Design review of the part shown in the three views and the two pictorial views. Dimensions are in mm from the part's minimum x, y and z. A direction names the side the tool comes from. Give positions to 0.01 mm unless a question says otherwise; leave off trailing zeros. Loops run counter-clockwise (first coordinate to the right, second up) from the corner with the lowest first, then second, coordinate; pieces in that order, holes last. Notation, with made-up numbers: M 10,11 L 15,11 A18 ccw 15,23 Z; hole C 37.25,22 d7. An arc over 180 degrees is marked long. Return JSON: item names as keys, results as strings. Group by question number.
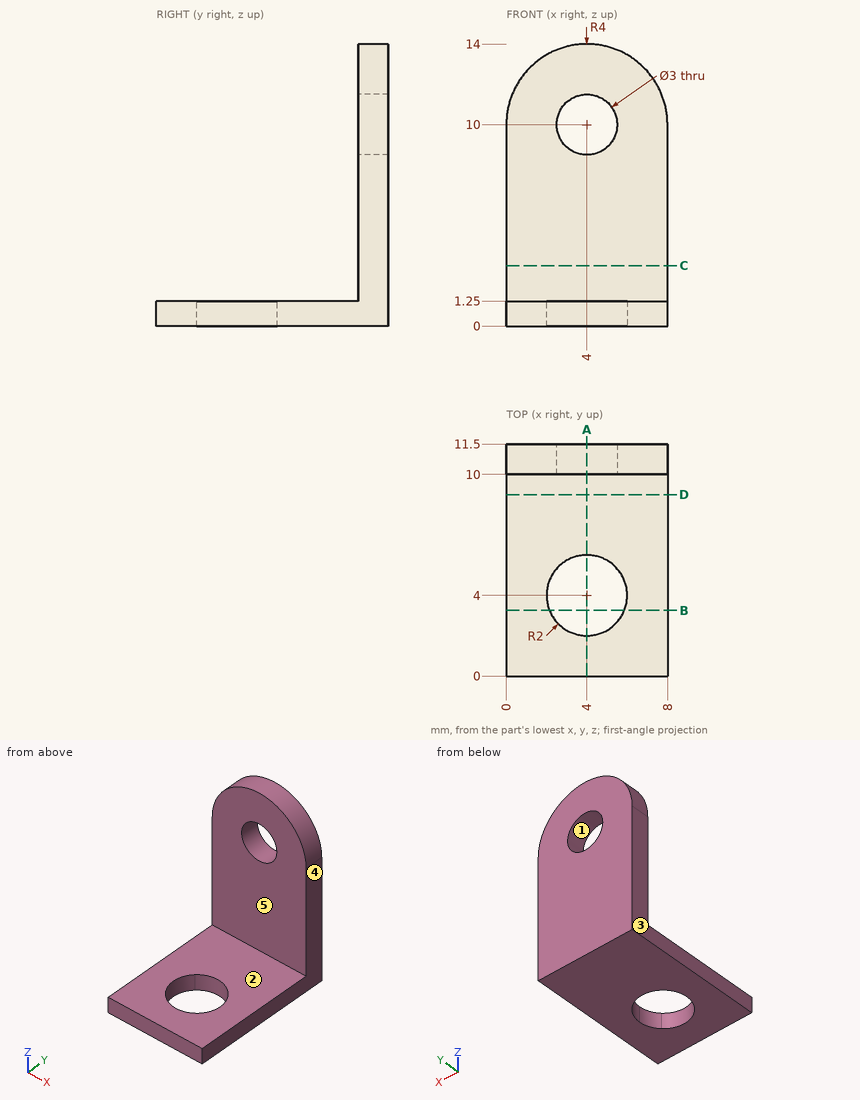
(1) Add section A-A (x = 4). Write out the cut boundary in (y, z).
(2) For probe 1 along Z at (x, y) = (4, 10.8); probe 2 along Z at (x, y) = (7.5, 0.75); probe 3 along Y at (x, z) = (2, 7), list the stretches that pass through material, from the lowest coordinate up.
(3) Add section C-C (z = 3). Write out the cut boundary in (x, y).
(4) Mouldability with a two-part tool opening along Z and no side actions: class the marked faces 1, 2 and 3 as released by +Z, released by -Z, zero draft, split by the parting line, or undercut.
(5) Add section D-D (y = 9). Write out the cut boundary in (x, z), and give its area (3 significant figures).
(6) For the marked faces 4 and 5, list the 3-axis set-ups (+Z, -Z, +X, -X, +Y, -Y) from which the entire face can be reached by the end or side of a thin tool; tool diameter is ignored.
(7) For pin 1 (2 mm diameter, centred on x = 3.5, y = 6, fed in from -Z); pin 2 (1.5 mm diameter, centred on x = 3.5, z = 7.5, fed in from -Y); pin 3 (4 mm diameter, centred on x = 4.5, y = 3, fed in from +Z), all flat-tipped, find the tip position at first contact; note any pin that passes through.
(8) Add section B-B (y = 3.25). Write out the cut boundary in (x, z).
Verdict:
{
 "1": {"outline": "M 0,0 L 2,0 L 2,1.25 L 0,1.25 Z; M 6,0 L 11.5,0 L 11.5,8.5 L 10,8.5 L 10,1.25 L 6,1.25 Z; M 10,11.5 L 11.5,11.5 L 11.5,14 L 10,14 Z"},
 "2": {"probe 1": "z = 0 to 8.5, 11.5 to 14", "probe 2": "z = 0 to 1.25", "probe 3": "y = 10 to 11.5"},
 "3": {"outline": "M 0,10 L 8,10 L 8,11.5 L 0,11.5 Z"},
 "4": {"face 1": "undercut", "face 2": "released by +Z", "face 3": "zero draft"},
 "5": {"outline": "M 0,0 L 8,0 L 8,1.25 L 0,1.25 Z", "area": "10.0 mm²"},
 "6": {"face 4": "+Z, -Z, +X, +Y, -Y", "face 5": "+Z, +X, -X, -Y"},
 "7": {"pin 1": "stops at z = 0", "pin 2": "stops at y = 10", "pin 3": "stops at z = 1.25"},
 "8": {"outline": "M 0,0 L 2.15,0 L 2.15,1.25 L 0,1.25 Z; M 5.85,0 L 8,0 L 8,1.25 L 5.85,1.25 Z"}
}
